```python
from build123d import *

# Parameters (mm, degrees)
F1_DEPTH = 25.4


# Not quite as in the source:
# - a feature names something its author has since deleted; it is built from what else it names


with BuildPart() as f1:
    # F0 (on Top) → F1 (new body)
    with BuildSketch(Plane.XY):
        with BuildLine():
            ThreePointArc((-6.920715507, 16.4643668374), (-6.4934894763, 14.6036920626), (-6.35, 12.7))
            Line((-6.35, 12.7), (6.35, 12.7))
            ThreePointArc((6.35, 12.7), (6.4934894763, 14.6036920626), (6.920715507, 16.4643668374))
            ThreePointArc((6.920715507, 16.4643668374), (0, 22.5641302142), (-6.920715507, 16.4643668374))
        make_face()
        with BuildLine():
            Line((6.35, 12.7), (-6.35, 12.7))
            ThreePointArc((-6.35, 12.7), (-10.0697438789, 3.7197438789), (-19.05, 0))
            ThreePointArc((-19.05, 0), (-10.0697438789, -3.7197438789), (-6.35, -12.7))
            Line((-6.35, -12.7), (6.35, -12.7))
            ThreePointArc((6.35, -12.7), (10.0697438789, -3.7197438789), (19.05, 0))
            ThreePointArc((19.05, 0), (10.0697438789, 3.7197438789), (6.35, 12.7))
        make_face()
        with BuildLine():
            Line((6.35, -12.7), (-6.35, -12.7))
            ThreePointArc((-6.35, -12.7), (-6.4956231596, -14.6177127391), (-6.9291530945, -16.4914469919))
            ThreePointArc((-6.9291530945, -16.4914469919), (0, -22.5949355663), (6.9291530945, -16.4914469919))
            ThreePointArc((6.9291530945, -16.4914469919), (6.4956231596, -14.6177127391), (6.35, -12.7))
        make_face()
    extrude(amount=F1_DEPTH)


solid = f1.part
```
Read the model definition and answer for the solid it produces. Units are mm, in the model's axes. Give positions to 0.01 mm unless a question says otherwise; leave off trailing zeros. Order: outer loops, then holes, each group sorted by start corner. A loop starts at its lowest first (then second) coordinate and runs counter-clockwise, first axis right, second up. Notation, with made-up numbers: (-34.75, 64.5) -> (-10.75, 64.5) arc R28 cw to (-10.75, 102.5) -> close; hole circle Ø1 at (-36.5, 63.5). An arc over 180 degrees is marked (long way). One line per item, written item: value. Start each with the question number.
(1) The part is cut by section A-A (z = 9.25). Determine the outline of the cut face in (x, y) (3 decimals).
(2) Flat-ended cylindrical pins translate along their axes: P1, Ø1, axis at x = 11, z = 15.5, coming from the -Y side; P2, Ø5, axis at y = -7.5, z = 17, coming from the +X side; P3, Ø10, axis at x = -14.5, z = 20.5, coming from the +Y side. Find the tip coordinate at first contact, or state that the pin passes through.
(3) The part is cut by section C-C (y = 15). Determine the outline of the cut face in (x, z).
(4) Straight lines are drawn through the part: L1, parallel to X at y = 9, z = 9.75; L2, parallel to Y at x = -4.5, z = 13.5; L3, parallel to Y at x = -15.5, z = 3.75. For each, find the intervals that lie inside material, in ascending order.
(5) The part is cut by section B-B (x = 8). Determine the outline of the cut face in (y, z), and give its area (3 significant figures).
Taken from the geometry:
1. outline: (-19.05, 0) arc R12.7 cw to (-6.929, -16.491) arc R6.985 ccw to (6.929, -16.491) arc R12.7 cw to (19.05, 0) arc R12.7 cw to (6.921, 16.464) arc R6.976 ccw to (-6.921, 16.464) arc R12.7 cw to start
2. P1: y = -3.31
2. P2: x = 8.95
2. P3: y = 4.33
3. outline: (-6.56, 0) -> (6.56, 0) -> (6.56, 25.4) -> (-6.56, 25.4) -> close
4. L1: -6.9 to 6.9
4. L2: -20.95 to 20.92
4. L3: -0.51 to 0.51
5. outline: (-6.44, 0) -> (6.44, 0) -> (6.44, 25.4) -> (-6.44, 25.4) -> close
5. area: 327 mm^2
